Design review of the part shown in the three views and the two pictorial views. Dimensions are in mm from the part's minimum x, y and z. A direction names the side the tool comes from. Coordinates: 2 decimals unless noted, no trailing zeros. Loops run counter-clockwise (first coordinate to the right, second up) from the corner with the lowest first, then second, coordinate; pieces in that order, holes last. Notation, with made-up numbers: (41, 22) -> (65, 22) arc R25 ccw to (65, 47) -> close; hole circle Ø6 at (24.5, -30). An arc over 180 degrees is marked (long way). Answer in a Markdown table with one row per item.
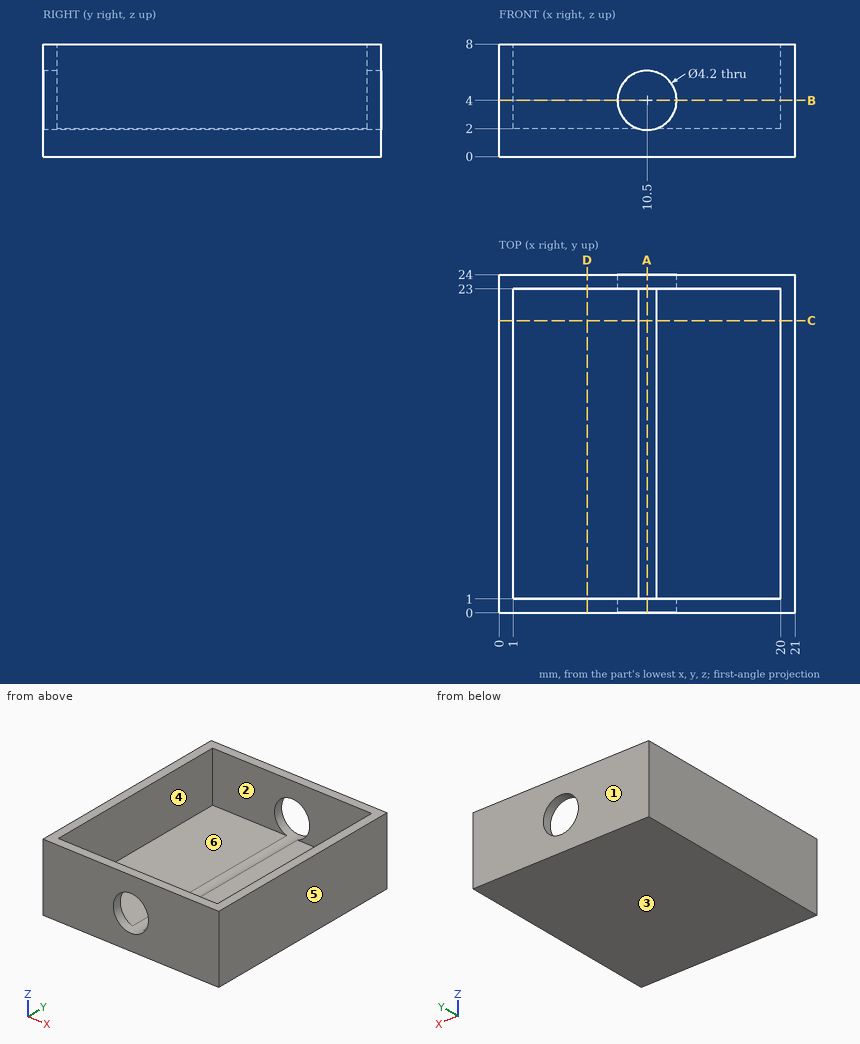
Item 1: Take a section at C-C, the plane y = 20.75. State the section outline as (x, z) points.
Worked answers:
| item | result |
|---|---|
| outline | (0, 0) -> (21, 0) -> (21, 8) -> (20, 8) -> (20, 2) -> (11.14, 2) arc R2.1 cw to (9.86, 2) -> (1, 2) -> (1, 8) -> (0, 8) -> close |
Item 2: For the marked faces 1 and 2, list the 3-axis set-ups (+Z, -Z, +X, -X, +Y, -Y) from which the entire face can be reached by the end or side of a thin tool; tool diameter is ignored.
Worked answers:
| item | result |
|---|---|
| face 1 | +Z, -Z, +X, -X, +Y |
| face 2 | +Z |
Item 3: Take a section at A-A, the plane x = 10.5. State the section outline as (y, z) points, and give its area (3 significant figures).
Worked answers:
| item | result |
|---|---|
| outline | (0, 0) -> (24, 0) -> (24, 1.9) -> (0, 1.9) -> close; (0, 6.1) -> (1, 6.1) -> (1, 8) -> (0, 8) -> close; (23, 6.1) -> (24, 6.1) -> (24, 8) -> (23, 8) -> close |
| area | 49.4 mm² |
Item 4: Insertion check: pin 1 (7 mm diameter, centred on x = 7.5, y = 12, fed in from +Z); pin 2 (1.5 mm diameter, centred on x = 4.5, y = 11, fed in from -Z). Each pin has a flat end and moves straight along its axis. Give the tip position at first contact, or say it passes through.
Worked answers:
| item | result |
|---|---|
| pin 1 | z = 2 |
| pin 2 | z = 0 |
Item 5: The part is to be moulded in two halves that separate along X. For the marked faces 3, 4, 5 and 6, say which applies: +X half, -X half, draft (parallel to the pull), parting line (faces both ways), or undercut.
Worked answers:
| item | result |
|---|---|
| face 3 | draft |
| face 4 | undercut |
| face 5 | +X half |
| face 6 | undercut |
Item 6: Take a section at B-B, the plane z = 4. State the section outline as (x, y) points.
Worked answers:
| item | result |
|---|---|
| outline | (0, 0) -> (8.4, 0) -> (8.4, 1) -> (1, 1) -> (1, 23) -> (8.4, 23) -> (8.4, 24) -> (0, 24) -> close; (12.6, 0) -> (21, 0) -> (21, 24) -> (12.6, 24) -> (12.6, 23) -> (20, 23) -> (20, 1) -> (12.6, 1) -> close |
Item 7: Take a section at D-D, the plane x = 6.25. State the section outline as (y, z) points.
Worked answers:
| item | result |
|---|---|
| outline | (0, 0) -> (24, 0) -> (24, 8) -> (23, 8) -> (23, 2) -> (1, 2) -> (1, 8) -> (0, 8) -> close |
Item 8: For L1, parallel to Y at x = 1.75, z = 3; L2, parallel to X at y = 18.75, z = 4; L3, parallel to Z at x = 13, y = 19, list the stretches that pass through material, from the lowest coordinate up.
Worked answers:
| item | result |
|---|---|
| L1 | 0 to 1, 23 to 24 |
| L2 | 0 to 1, 20 to 21 |
| L3 | 0 to 2 |
